Autodesk Inventor part; units mm, degrees
ref_plane "YZ Plane" through (0, 0, 0) normal (1, 0, 0) x (0, 1, 0)
ref_plane "XZ Plane" through (0, 0, 0) normal (0, 1, 0) x (-1, 0, 0)
ref_plane "XY Plane" through (0, 0, 0) normal (0, 0, 1) x (1, 0, 0)
sketch "Sketch1" plane through (0, 0, 0) normal (1, 0, 0) x (0, 1, 0)
  line L0 (0, 0) -> (0, -101.6)
  arc A0 (0, -101.6) -> (406.4, -508) centre (406.4, -101.6) ccw
  line L1 (406.4, -508) -> (508, -508)
  dimension "bendAngle" = 90
  dimension "centerlineRadius" = 406.4
  dimension "tangentLength" = 101.6
sketch "Sketch2" plane through (0, 0, 0) normal (0, 0, 1) x (1, 0, 0)
  circle A0 centre (0, 0) radius 50.8
  circle A1 centre (0, 0) radius 44.45
  dimension "outerDiameter" = 101.6
  dimension "wallThickness" = 6.35
sweep "Sweep1" add profiles "Sketch2" path "Sketch1"
properties part number "Tube Bend"
Source: CAD feature listing. Evaluate the final solid. Frame: model axes, mm. A direction names the side the tool comes from. Round coordinates to 2 decimals unless told otherwise and drop trailing zeros. Loops run counter-clockwise (first coordinate to the right, second up) from the corner with the lowest first, then second, coordinate; pieces in that order, holes last. Notation, with made-up numbers: (-1, -28.75) - (44, -28.75) arc R24 ccw to (44, 1.25) - close; hole circle Ø5 at (7, 68). An arc over 180 degrees is marked (long way). Write item = value, one per line. Start each with the question number.
Item 1: Section query A-A on x = 0. Output: boundary loops of the cut face in (y, z), plus the area to 3 significant figures.
Item 2: Mould query, pull axis Y, two halves, no side actions, for faces 1 (the face through (-45, 508, -508)), 2 (the face through (42.397, -13.352, -51.511)), 3 (the face through (-11.012, 49.592, -51.511)), 4 (the face through (-11.012, 457.911, -458.408)). Classes: released by +Y, released by -Y, zero draft, split by the parting line, or undercut.
Item 3: First-contact query: pin 1 Ø4 at (y, z) = (42, -269) entering from +X; pin 2 Ø6 at (x, y) = (-32, 21) entering from -Z; pin 3 Ø8 at (x, z) = (40, -404) entering from -Y. Flat tips, straight axial feed; report the tip coordinate or a pass-through.
Item 4: Material intervals for line 1 (X direction, y = 477, z = -508); line 2 (Z direction, x = 0, y = 451.5), sorted ascending.
Item 5: Section query C-C on y = 470.5. Output: boundary loops of the cut face in (x, z).
Item 6: Reachability of faces 5 (the face through (0, -45, 0)), 6 (the face through (-9.6, 457.9, -464.6)) from +Z, -Z, +X, -X, +Y, -Y: full face, straight path, thin tool, end or side. Return the list, or none.
Item 7: Section query B-B on x = 34.5. Output: boundary loops of the cut face in (y, z).
Results list:
q1.outline = (-50.8, -101.6) arc R457.2 ccw to (406.4, -558.8) - (508, -558.8) - (508, -552.45) - (406.4, -552.45) arc R450.85 cw to (-44.45, -101.6) - (-44.45, 0) - (-50.8, 0) - close; (44.45, -101.6) arc R361.95 ccw to (406.4, -463.55) - (508, -463.55) - (508, -457.2) - (406.4, -457.2) arc R355.6 cw to (50.8, -101.6) - (50.8, 0) - (44.45, 0) - close
q1.area = 10,700 mm²
q2.face_1 = released by +Y
q2.face_2 = undercut
q2.face_3 = split by the parting line
q2.face_4 = zero draft
q3.pin_1 = 50.69
q3.pin_2 = -332.57
q3.pin_3 = 82.58
q4.line_1 = -50.8 to -44.45, 44.45 to 50.8
q4.line_2 = -558.8 to -552.45, -463.55 to -457.2
q5.outline = circle Ø101.6 at (0, -508); hole circle Ø88.9 at (0, -508)
q6.face_5 = +Z, +X, -X, +Y, -Y
q6.face_6 = +Y
q7.outline = (-37.29, -101.6) arc R443.69 ccw to (406.4, -545.29) - (508, -545.29) - (508, -536.03) - (406.4, -536.03) arc R434.43 cw to (-28.03, -101.6) - (-28.03, 0) - (-37.29, 0) - close; (28.03, -101.6) arc R378.37 ccw to (406.4, -479.97) - (508, -479.97) - (508, -470.71) - (406.4, -470.71) arc R369.11 cw to (37.29, -101.6) - (37.29, 0) - (28.03, 0) - close
